Could you check a few things on this model? Use its own coordinates, in mm. A direction names the side the tool comes from. Coordinates: 2 decimals unless noted, no trailing zeros. Write each loop counter-clockwise with the first axis right and the second up, starting at its lowest first coordinate (ties: lowest second). Pieces come first, ordered by that corner, then holes. Notation, with made-up numbers: M -2,52 L 3,52 A7 cw 3,63 Z; hole C 85,-27.5 d1. An arc over 180 degrees is marked long. Write item = value, one per line.
Autodesk Inventor part; units mm, degrees
ref_plane "YZ Plane" through (0, 0, 0) normal (1, 0, 0) x (0, 1, 0)
ref_plane "XZ Plane" through (0, 0, 0) normal (0, 1, 0) x (-1, 0, 0)
ref_plane "XY Plane" through (0, 0, 0) normal (0, 0, 1) x (1, 0, 0)
sketch "Sketch1" plane through (0, 0, 0) normal (0, 0, 1) x (1, 0, 0)
  line L0 (-28.5, 28.5) -> (28.5, 28.5)
  line L1 (28.5, 28.5) -> (28.5, -28.5)
  line L2 (28.5, -28.5) -> (-28.5, -28.5)
  line L3 (-28.5, -28.5) -> (-28.5, 28.5)
  line L4 (-15, 15) -> (15, 15)
  line L5 (15, 15) -> (15, -15)
  line L6 (15, -15) -> (-15, -15)
  line L7 (-15, -15) -> (-15, 15)
  line L8 (-18.5, 28.5) -> (-18.5, 18.5)
  line L9 (-18.5, 18.5) -> (-28.5, 18.5)
  line L10 (18.5, 28.5) -> (18.5, 18.5)
  line L11 (18.5, 18.5) -> (28.5, 18.5)
  line L12 (28.5, -18.5) -> (18.5, -18.5)
  line L13 (18.5, -18.5) -> (18.5, -28.5)
  line L14 (-28.5, -18.5) -> (-18.5, -18.5)
  line L15 (-18.5, -18.5) -> (-18.5, -28.5)
  line L16 (-18.5, 28.5) -> (18.5, 28.5)
  line L17 (28.5, 18.5) -> (28.5, -18.5)
  line L18 (18.5, -28.5) -> (-18.5, -28.5)
  line L19 (-28.5, -18.5) -> (-28.5, 18.5)
  point P0 (0, 0)
  dimension "d0" = 28.5
  dimension "d1" = 28.5
  dimension "d2" = 57
  dimension "d3" = 57
  dimension "d4" = 30
  dimension "d5" = 30
  dimension "d6" = 15
  dimension "d7" = 15
  dimension "d8" = 10
  dimension "d9" = 10
  dimension "d10" = 10
  dimension "d11" = 10
  dimension "d12" = 10
  dimension "d13" = 10
  dimension "d14" = 10
extrude "Extrusion1" add sketch "Sketch1" along normal mid plane 65 contours L0 L10 L11 L1 L12 L13 L2 L15 L14 L3 L9 L8
sketch "Sketch2" plane through (28.5, -18.5, 32.5) normal (1, 0, 0) x (0, 0, -1)
  line L0 (65, 33.5) -> (65, 3.5)
  line L1 (65, 18.5) -> (65, 28.5)
  line L2 (65, 28.5) -> (50, 28.5)
  line L3 (50, 28.5) -> (50, 8.5)
  line L4 (50, 8.5) -> (65, 8.5)
  point P0 (32.5, 18.5)
  dimension "d17" = 10
  dimension "d20" = 15
  dimension "d22" = 20
extrude "Extrusion2" add sketch "Sketch2" along normal blind 7
chamfer "Chamfer1" distance 2 angle 45 4 edges at (35.5, 10, -25) (35.5, 0, -32.5) (35.5, -10, -25) (35.5, 0, -17.5)
properties part number "MotorBody"
Item 1: If I drill on line 1 along Y through (x, z) = (4.5, 4); line 2 along X through (y, z) = (5, -22.5), over which ranges is the centre line in solid material (lowest first)?
Numbers:
line_1 = -28.5 to -15, 15 to 28.5
line_2 = -28.5 to -15, 15 to 35.5
Item 2: Imagine slicing it at B-B (x = 8). Write out the boundary of the cut face in (y, z).
Numbers:
outline = M -28.5,-32.5 L -15,-32.5 L -15,32.5 L -28.5,32.5 Z; M 15,-32.5 L 28.5,-32.5 L 28.5,32.5 L 15,32.5 Z
Item 3: If we mould it in two halves opening along X, with no side actions, what happens to faces 1 (the face through (-23, 18.5, 0)), 2 (the face through (-18.5, -23, 0)), 3 (the face through (0, -15, 0))? For each: pulls with the +X half, pulls with the -X half, needs draft (parallel to the pull), parting line crosses it, or undercut.
Numbers:
face_1 = needs draft
face_2 = pulls with the -X half
face_3 = undercut
Item 4: Imagine slicing it at A-A (y = -1). Write out the boundary of the cut face in (x, z).
Numbers:
outline = M -28.5,-32.5 L -15,-32.5 L -15,32.5 L -28.5,32.5 Z; M 15,-32.5 L 33.5,-32.5 L 35.5,-30.5 L 35.5,-19.5 L 33.5,-17.5 L 28.5,-17.5 L 28.5,32.5 L 15,32.5 Z
Item 5: For faces 4 (the face through (35.5, 0, -25)), 5 (the face through (31, 10, -25)), 6 (the face through (-18.5, 24, 0)), 7 (the face through (-24, -18.5, 0)), 8 (the face through (0, 15, 0)), which set-ups out of +Z, -Z, +X, -X, +Y, -Y let a thin tool reach every point of the face, with its end or its side?
Numbers:
face_4 = +Z, -Z, +X, +Y, -Y
face_5 = +Z, -Z, +X, +Y
face_6 = +Z, -Z, -X, +Y
face_7 = +Z, -Z, -X, -Y
face_8 = +Z, -Z
Item 6: I'm going to push flat-ended pins straight in: P1, Ø3, axis at y = -21.5, z = -14.5, coming from the +X side; P2, Ø4, axis at x = 30, y = -4, coming from the +Z side; P3, Ø2, axis at y = 1, z = 8.5, coming from the +X side; P4, Ø11, axis at x = -24.5, z = 5, coming from the +Y side. Where does each tip first touch, or does it pass through?
Numbers:
P1 = 18.5
P2 = 32.5
P3 = 28.5
P4 = 18.5
Item 7: Imagine slicing it at D-D (y = 16). Write out the boundary of the cut face in (x, z), and give its area (4 significant figures).
Numbers:
outline = M -28.5,-32.5 L 28.5,-32.5 L 28.5,32.5 L -28.5,32.5 Z
area = 3,705 mm²
Item 8: Imagine slicing it at C-C (z = 28.5). Write out the boundary of the cut face in (x, y).
Numbers:
outline = M -28.5,-18.5 L -18.5,-18.5 L -18.5,-28.5 L 18.5,-28.5 L 18.5,-18.5 L 28.5,-18.5 L 28.5,18.5 L 18.5,18.5 L 18.5,28.5 L -18.5,28.5 L -18.5,18.5 L -28.5,18.5 Z; hole M -15,-15 L 15,-15 L 15,15 L -15,15 Z
